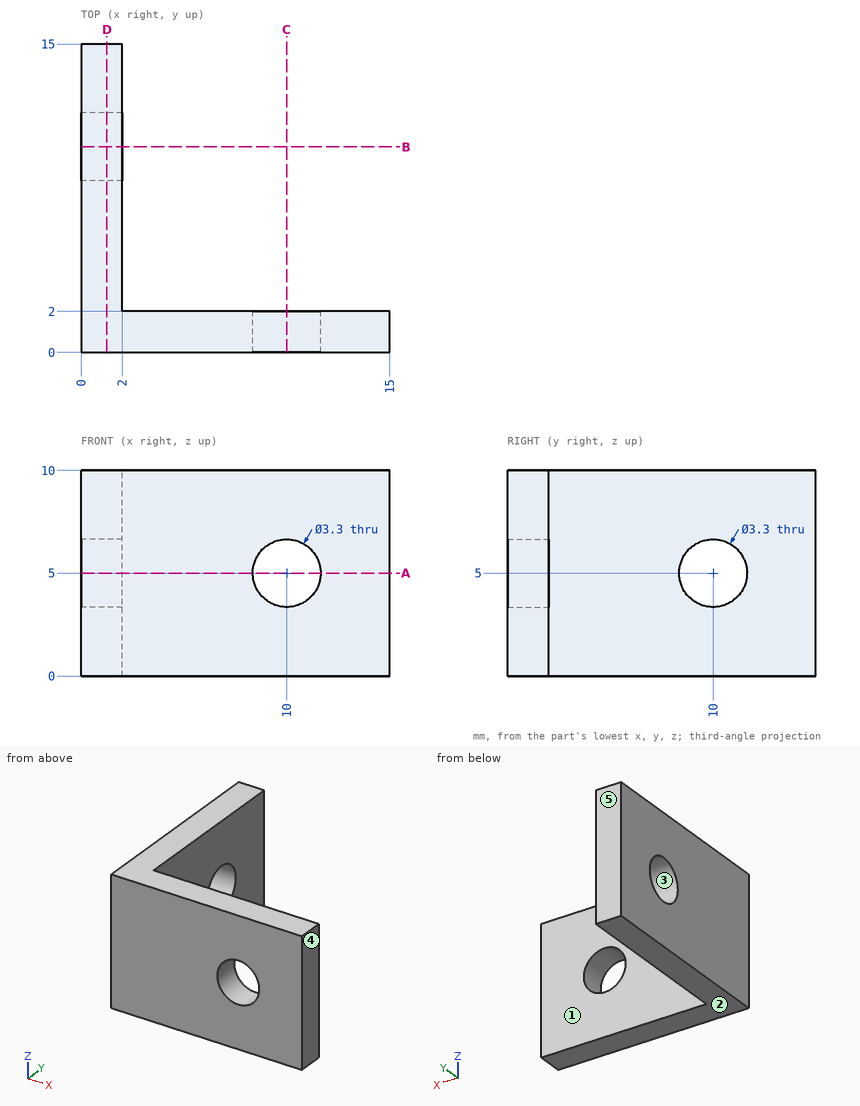
Design review of the part shown in the three views and the two pictorial views. Dimensions are in mm from the part's minimum x, y and z. A direction names the side the tool comes from. Round coordinates to 2 decimals unless told otherwise and drop trailing zeros. Write each loop counter-clockwise with the first axis right and the second up, starting at its lowest first coordinate (ties: lowest second). Pieces come first, ordered by that corner, then holes.
1) Mouldability with a two-part tool opening along Y and no side actions: class the marked faces 3, 4 and 5 as +Y half, -Y half, draft (parallel to the pull), parting line (faces both ways), or undercut.
Answer below:
face 3: undercut
face 4: draft
face 5: +Y half
2) Machinability: for the marked faces 1 and 2, which of the approach directions +Z, -Z, +X, -X, +Y, -Y give a long, thin tool a straight path to every point of the face, cutting with its end or side? Answer none if there is none.
Answer below:
face 1: +Z, -Z, +X, +Y
face 2: -Z, +X, -X, +Y, -Y
3) Insertion check: pin 1 Ø5 at (x, z) = (7.5, 8) entering from +Y; pin 2 Ø2.5 at (y, z) = (10, 5) entering from -X; pin 3 Ø1 at (y, z) = (7, 6) entering from +X. Each pin has a flat end and moves straight along its axis. Give the tip position at first contact, or say it passes through.
Answer below:
pin 1: stops at y = 2
pin 2: passes through
pin 3: stops at x = 2
4) For line 1 along Z through (x, y) = (1.25, 10); line 2 along Y through (x, z) = (0.85, 5); line 3 along Y through (x, z) = (12.25, 8.25), list the stretches that pass through material, from the lowest coordinate up.
Answer below:
line 1: z = 0 to 3.35, 6.65 to 10
line 2: y = 0 to 8.35, 11.65 to 15
line 3: y = 0 to 2
5) Take a section at B-B on y = 10. Give the boundary of the cut face in (x, z).
Answer below:
outline: (0, 0) - (2, 0) - (2, 3.35) - (0, 3.35) - close; (0, 6.65) - (2, 6.65) - (2, 10) - (0, 10) - close
6) Take a section at D-D on x = 1.25. Give the boundary of the cut face in (y, z).
Answer below:
outline: (0, 0) - (15, 0) - (15, 10) - (0, 10) - close; hole circle Ø3.3 at (10, 5)
7) Take a section at A-A on z = 5. Give the boundary of the cut face in (x, y).
Answer below:
outline: (0, 0) - (8.35, 0) - (8.35, 2) - (2, 2) - (2, 8.35) - (0, 8.35) - close; (0, 11.65) - (2, 11.65) - (2, 15) - (0, 15) - close; (11.65, 0) - (15, 0) - (15, 2) - (11.65, 2) - close
